Source: CAD feature listing. Evaluate the final solid. Frame: model axes, mm. A direction names the side the tool comes from. Coordinates: 2 decimals unless noted, no trailing zeros. Order: outer loops, then holes, each group sorted by start corner. A loop starts at its lowest first (then second) coordinate and runs counter-clockwise, first axis right, second up.
```python
from build123d import *

# Parameters (mm, degrees)
F1_DEPTH = 25


with BuildPart() as f1:
    # F0 (on Front) → F1 (new body)
    with BuildSketch(Plane.XZ):
        with BuildLine():
            Line((103.990591, -245.581819), (103.990591, -275.581819))
            Line((103.990591, -275.581819), (353.990591, -275.581819))
            Line((353.990591, -275.581819), (353.990591, -245.581819))
            ThreePointArc((353.990591, -245.581819), (348.132727, -231.439684), (333.990591, -225.581819))
            Line((333.990591, -225.581819), (253.990591, -225.581819))
            ThreePointArc((253.990591, -225.581819), (246.919523, -222.652887), (243.990591, -215.581819))
            Line((243.990591, -215.581819), (243.990591, -110.581819))
            ThreePointArc((243.990591, -110.581819), (242.526125, -107.046285), (238.990591, -105.581819))
            Line((238.990591, -105.581819), (198.990591, -105.581819))
            ThreePointArc((198.990591, -105.581819), (195.455057, -107.046285), (193.990591, -110.581819))
            Line((193.990591, -110.581819), (193.990591, -215.581819))
            ThreePointArc((193.990591, -215.581819), (191.061659, -222.652887), (183.990591, -225.581819))
            Line((183.990591, -225.581819), (123.990591, -225.581819))
            ThreePointArc((123.990591, -225.581819), (109.848456, -231.439684), (103.990591, -245.581819))
        make_face()
    extrude(amount=F1_DEPTH)


solid = f1.part
```
Q1. Material intervals for line 1 along Z through (x, y) = (281, -12.5); line 2 along X through (y, z) = (-18, -120); line 3 along Z through (x, y) = (242, -10.5), sorted ascending.
Solutions:
line 1: z = -275.58 to -225.58
line 2: x = 193.99 to 243.99
line 3: z = -275.58 to -106.59
Q2. Section query B-B on x = 302. Output: boundary loops of the cut face in (y, z).
Solutions:
outline: (-25, -275.58) - (0, -275.58) - (0, -225.58) - (-25, -225.58) - close
Q3. Pin query (flat end, axial travel): P1, Ø5, axis at x = 296, y = -20, coming from the +Z side; P2, Ø1.5, axis at y = -17, z = -133.5, coming from the +X side. Return the tip coordinate at first contact, or that it passes through.
Solutions:
P1: stops at z = -225.58
P2: stops at x = 243.99
Q4. Section query A-A on y = -22. Output: boundary loops of the cut face in (x, z).
Solutions:
outline: (103.99, -275.58) - (353.99, -275.58) - (353.99, -245.58) arc R20 ccw to (333.99, -225.58) - (253.99, -225.58) arc R10 cw to (243.99, -215.58) - (243.99, -110.58) arc R5 ccw to (238.99, -105.58) - (198.99, -105.58) arc R5 ccw to (193.99, -110.58) - (193.99, -215.58) arc R10 cw to (183.99, -225.58) - (123.99, -225.58) arc R20 ccw to (103.99, -245.58) - close
Q5. Section query C-C on z = -179. Output: boundary loops of the cut face in (x, y), plus the area to 3 significant figures.
Solutions:
outline: (193.99, -25) - (243.99, -25) - (243.99, 0) - (193.99, 0) - close
area: 1,250 mm2
Q6. Set-up query: faces 1 (the flat face through (154, -12, -225.582)), 2 (the flat face through (103.991, -12, -260)), 3 (the flat face through (243.991, -12, -164)). Return all of +Z, -Z, +X, -X, +Y, -Y with unobstructed straight access to the full face (end or side cutting, diameter ignored); none if empty.
Solutions:
face 1: +Z, -X, +Y, -Y
face 2: +Z, -Z, -X, +Y, -Y
face 3: +Z, +X, +Y, -Y
